```python
from build123d import *

# Parameters (mm, degrees)
SKETCH2_W           = 42.6
SKETCH2_H           = 21.95
BOSS_EXTRUDE1_DEPTH = 7.2
FILLET1_R           = 3
SKETCH3_W           = 4.07
SKETCH3_H           = 13.25
CUT_EXTRUDE1_DEPTH  = 5.2
BOSS_EXTRUDE2_DEPTH = 5.2
BOSS_EXTRUDE3_DEPTH = 4.2


with BuildPart() as part:
    # Sketch2 → Boss-Extrude1 (new body)
    with BuildSketch(Plane.XY):
        Rectangle(SKETCH2_W, SKETCH2_H)
    extrude(amount=BOSS_EXTRUDE1_DEPTH)

    # Fillet1
    fillet1_edges = [part.edges().sort_by_distance(p)[0] for p in [
        (-21.3, 10.975, 3.6),
        (21.3, 10.975, 3.6),
        (21.3, -10.975, 3.6),
        (-21.3, -10.975, 3.6),
    ]]
    fillet(fillet1_edges, radius=FILLET1_R)

    # Sketch3 → Cut-Extrude1 (cut)
    with BuildSketch(Plane(origin=(0, 0, 0), x_dir=(-1, 0, 0), z_dir=(0, 0, -1))):
        with Locations((-19.265, 0)):
            Rectangle(SKETCH3_W, SKETCH3_H)
    extrude(amount=-CUT_EXTRUDE1_DEPTH, mode=Mode.SUBTRACT)

    # Sketch4 → Boss-Extrude2 (add)
    with BuildSketch(Plane(origin=(0, 0, 5.2), x_dir=(-1, 0, 0), z_dir=(0, 0, -1))):
        Polygon((-20.15, 4.925), (-20.15, -4.925), (-18.4, -4.925), (-18.4, -3.815), (-19.11, -3.815), (-19.11, -0.555), (-18.4, -0.555), (-18.4, 0.555), (-19.11, 0.555), (-19.11, 3.815), (-18.4, 3.815), (-18.4, 4.925), align=None)
    extrude(amount=BOSS_EXTRUDE2_DEPTH)

    # Sketch5 → Boss-Extrude3 (add)
    with BuildSketch(Plane(origin=(0, 0, 5.2), x_dir=(-1, 0, 0), z_dir=(0, 0, -1))):
        Polygon((-21.3, 6.625), (-21.3, -6.625), (-19.9, -6.625), (-19.9, -4.925), (-20.15, -4.925), (-20.15, 4.925), (-19.9, 4.925), (-19.9, 6.625), align=None)
    extrude(amount=BOSS_EXTRUDE3_DEPTH)


solid = part.part
```
Here's how the part is built. I have some questions about the finished solid (model axes, mm). A direction names the side the tool comes from. Round coordinates to 2 decimals unless told otherwise and drop trailing zeros. Write each loop counter-clockwise with the first axis right and the second up, starting at its lowest first coordinate (ties: lowest second). Pieces come first, ordered by that corner, then holes.
Q1. If we section it at B-B on y = 1.25: Write out the boundary of the cut face in (x, z).
Q2. If we section it at A-A on z = 2: Write out the boundary of the cut face in (x, y) (3 decimals), plus the area to 3 significant figures.
Q3. Which directions (+Z, -Z, +X, -X, +Y, -Y) give clear straight access to the entire face, cutting with the end or side of a thin tool? Please do faces 1 (the cylindrical face through (-20.445, 10.073, 3.65)), 2 (the flat face through (19.9, -6, 3)).
Q4. Will these pins go through, and if not, where does the flat tip stop? P1, Ø0.8, axis at y = 2, z = 0.5, coming from the +X side; P2, Ø0.8, axis at x = 19, z = 4, coming from the +Y side.
Q5. If we section it at C-C on y = -5.75: Write out the boundary of the cut face in (x, z).
Q6. Please list where these lines run through material, in increasing order: probe 1 along X at (y, z) = (-5, 3); probe 2 along X at (y, z) = (4.5, 3.5); probe 3 along Y at (x, z) = (19, 1.75) (3 decimals).
Q7. If we mould it in two halves opening along X, with no side actions, what happens to faces 3 (the flat face through (17.23, 0, 3)), 4 (the flat face through (21.3, 0, 4)), 5 (the flat face through (0, 0, 0)), 6 (the flat face through (-21.3, 0, 4))? For each: +X half, -X half, draft (parallel to the pull), parting line (faces both ways), or undercut.
Answer below:
1. outline: (-21.3, 0) - (17.23, 0) - (17.23, 5.2) - (19.11, 5.2) - (19.11, 0) - (20.15, 0) - (20.15, 1) - (21.3, 1) - (21.3, 7.2) - (-21.3, 7.2) - close
2. outline: (-21.3, -7.975) arc R3 ccw to (-18.3, -10.975) - (18.3, -10.975) arc R3 ccw to (21.3, -7.975) - (21.3, 7.975) arc R3 ccw to (18.3, 10.975) - (-18.3, 10.975) arc R3 ccw to (-21.3, 7.975) - close; hole (17.23, -6.625) - (19.9, -6.625) - (19.9, -4.925) - (18.4, -4.925) - (18.4, -3.815) - (19.11, -3.815) - (19.11, -0.555) - (18.4, -0.555) - (18.4, 0.555) - (19.11, 0.555) - (19.11, 3.815) - (18.4, 3.815) - (18.4, 4.925) - (19.9, 4.925) - (19.9, 6.625) - (17.23, 6.625) - close
2. area: 902 mm2
3. face 1: +Z, -Z, -X, +Y
3. face 2: -Z
4. P1: stops at x = 20.15
4. P2: stops at y = 10.96
5. outline: (-21.3, 0) - (17.23, 0) - (17.23, 5.2) - (19.9, 5.2) - (19.9, 1) - (21.3, 1) - (21.3, 7.2) - (-21.3, 7.2) - close
6. probe 1: x = -21.3 to 17.23, 19.9 to 21.3
6. probe 2: x = -21.3 to 17.23, 18.4 to 21.3
6. probe 3: y = -10.892 to -6.625, -4.925 to -3.815, -0.555 to 0.555, 3.815 to 4.925, 6.625 to 10.892
7. face 3: undercut
7. face 4: +X half
7. face 5: draft
7. face 6: -X half
